```python
from build123d import *

# Parameters (mm, degrees)
SKETCH1_W           = 30
SKETCH1_H           = 150
BOSS_EXTRUDE2_DEPTH = 23
SKETCH3_W           = 28
SKETCH3_H           = 19
CUT_EXTRUDE1_DEPTH  = 193
SKETCH7_W           = 1.99467658
SKETCH7_H           = 23
BOSS_EXTRUDE4_DEPTH = 20
CUT_EXTRUDE2_DEPTH  = 20
SKETCH9_W           = 30
SKETCH9_H           = 10
BOSS_EXTRUDE5_DEPTH = 20
SKETCH11_R          = 2.5
CUT_EXTRUDE4_DEPTH  = 10
CUT_EXTRUDE5_DEPTH  = 30
FILLET1_R           = 10
SKETCH13_R          = 2.543230184
CUT_EXTRUDE6_DEPTH  = 30
FILLET2_R           = 10
FILLET3_R           = 10
FILLET4_R           = 2


with BuildPart() as part:
    # Sketch1 → Boss-Extrude2 (new body)
    with BuildSketch(Plane.XY):
        with Locations((15, 75)):
            Rectangle(SKETCH1_W, SKETCH1_H)
    extrude(amount=BOSS_EXTRUDE2_DEPTH)

    # Sketch3 → Cut-Extrude1 (cut)
    with BuildSketch(Plane(origin=(0, 150, 0), x_dir=(1, 0, 0), z_dir=(0, 1, 0))):
        with Locations((14, -11.5)):
            Rectangle(SKETCH3_W, SKETCH3_H)
    extrude(amount=-CUT_EXTRUDE1_DEPTH, mode=Mode.SUBTRACT)

    # Sketch7 → Boss-Extrude4 (add)
    with BuildSketch(Plane(origin=(0, 150, 0), x_dir=(1, 0, 0), z_dir=(0, 1, 0))):
        with Locations((29.00266171, -11.5)):
            Rectangle(SKETCH7_W, SKETCH7_H)
    extrude(amount=BOSS_EXTRUDE4_DEPTH)

    # Sketch8 → Cut-Extrude2 (cut)
    with BuildSketch(Plane(origin=(30, 0, 0), x_dir=(0, 0, -1), z_dir=(1, 0, 0))):
        with BuildLine():
            ThreePointArc((-11.5, 78), (-14.5, 75), (-11.5, 72))
            Line((-11.5, 72), (-11.5, 78))
        make_face()
        with BuildLine():
            Line((-11.5, 78), (-11.5, 72))
            ThreePointArc((-11.5, 72), (-9.378679656, 72.878679656), (-8.5, 75))
            ThreePointArc((-8.5, 75), (-9.378679656, 77.121320344), (-11.5, 78))
        make_face()
        with BuildLine():
            ThreePointArc((-13.763816566, 158.031463855), (-11.5, 157), (-9.236183434, 158.031463855))
            Line((-9.236183434, 158.031463855), (-11.5, 160))
            Line((-11.5, 160), (-13.763816566, 158.031463855))
        make_face()
        with BuildLine():
            Line((-11.5, 160), (-9.236183434, 158.031463855))
            ThreePointArc((-9.236183434, 158.031463855), (-8.690066754, 158.94915503), (-8.5, 160))
            ThreePointArc((-8.5, 160), (-8.690066754, 161.05084497), (-9.236183434, 161.968536145))
            Line((-9.236183434, 161.968536145), (-11.5, 160))
        make_face()
        with BuildLine():
            ThreePointArc((-13.763816566, 161.968536145), (-14.5, 160), (-13.763816566, 158.031463855))
            Line((-13.763816566, 158.031463855), (-11.5, 160))
            Line((-11.5, 160), (-13.763816566, 161.968536145))
        make_face()
        with BuildLine():
            Line((-11.5, 160), (-9.236183434, 161.968536145))
            ThreePointArc((-9.236183434, 161.968536145), (-11.5, 163), (-13.763816566, 161.968536145))
            Line((-13.763816566, 161.968536145), (-11.5, 160))
        make_face()
    extrude(amount=-CUT_EXTRUDE2_DEPTH, mode=Mode.SUBTRACT)

    # Sketch9 → Boss-Extrude5 (add)
    with BuildSketch(Plane.XY.offset(23)):
        with Locations((15, 75)):
            Rectangle(SKETCH9_W, SKETCH9_H)
    extrude(amount=BOSS_EXTRUDE5_DEPTH)

    # Sketch11 → Cut-Extrude4 (cut)
    with BuildSketch(Plane.XY.offset(23)):
        with Locations((7.001330855, 130)):
            Circle(SKETCH11_R)
        with Locations((7.5, 20)):
            Circle(SKETCH11_R)
    extrude(amount=-CUT_EXTRUDE4_DEPTH, mode=Mode.SUBTRACT)

    # Sketch12 → Cut-Extrude5 (cut)
    with BuildSketch(Plane.XY.offset(23)):
        Polygon((27.698367508, 150), (0, 150), (0, 140), align=None)
        Polygon((0, 0), (0, 10), (27.698367508, 0), align=None)
    extrude(amount=-CUT_EXTRUDE5_DEPTH, mode=Mode.SUBTRACT)

    # Fillet1
    fillet1_edges = [part.edges().sort_by_distance(p)[0] for p in [
        (0, 140, 1),
        (0, 10, 22),
        (0, 10, 1),
        (0, 140, 22),
    ]]
    fillet(fillet1_edges, radius=FILLET1_R)

    # Sketch13 → Cut-Extrude6 (cut)
    with BuildSketch(Plane.XY.offset(23)):
        with Locations((7.5, 20)):
            Circle(SKETCH13_R)
    extrude(amount=-CUT_EXTRUDE6_DEPTH, mode=Mode.SUBTRACT)

    # Fillet2
    fillet2_edges = [part.edges().sort_by_distance(p)[0] for p in [
        (0, 75, 43),
        (30, 75, 43),
    ]]
    fillet(fillet2_edges, radius=FILLET2_R)

    # Fillet3
    fillet3_edges = [part.edges().sort_by_distance(p)[0] for p in [
        (29.00266171, 170, 23),
        (29.00266171, 170, 0),
    ]]
    fillet(fillet3_edges, radius=FILLET3_R)

    # Fillet4
    fillet4_edges = [part.edges().sort_by_distance(p)[0] for p in [
        (30, 0, 11.5),
    ]]
    fillet(fillet4_edges, radius=FILLET4_R - 0.0001)  # a hair under: the kernel refuses the full size


solid = part.part
```
Work out the finished part from the listing and answer in its coordinate system (mm). A direction names the side the tool comes from. Coordinates: 2 decimals unless noted, no trailing zeros. Loops run counter-clockwise (first coordinate to the right, second up) from the corner with the lowest first, then second, coordinate; pieces in that order, holes last.
1) Section B-B (x = 23) is taken. Give the vertices of the cut face in (y, z).
Results:
outline: (1.7, 0) - (148.3, 0) - (148.3, 2) - (1.7, 2) - close; (1.7, 21) - (148.3, 21) - (148.3, 23) - (80, 23) - (80, 42.54) - (70, 42.54) - (70, 23) - (1.7, 23) - close
2) For faces 1 (the flat face through (14, 76, 21)), 2 (the cylindrical face through (2.85, 75.07, 39.99)), 3 (the flat face through (17.004, 3.861, 1.014)), 4 (the flat face through (15, 111, 23)), 5 (the flat face through (28.005, 158, 9)), determine the directions among +Z, -Z, +X, -X, +Y, -Y from which every point of the face is accessible in a straight line to the end or side of a thin tool.
Results:
face 1: -X, +Y, -Y
face 2: +Z, -X, +Y, -Y
face 3: +Z, -Z, -X, -Y
face 4: +Z, +X, -X, +Y
face 5: +Z, -Z, -X, +Y
3) Flat-ended cylindrical pins translate along their axes: pin 1 (16 mm diameter, centred on x = 16.5, z = 32.5, fed in from +Y); pin 2 (10 mm diameter, centred on x = 17, z = 18, fed in from +Y); pin 3 (6 mm diameter, centred on x = 17, y = 31.5, fed in from -Z); pin 4 (16 mm diameter, centred on y = 163.5, z = 11, fed in from -X). Find the tip coordinate at first contact, or state that the pin passes through.
Results:
pin 1: stops at y = 80
pin 2: stops at y = 147.58
pin 3: stops at z = 0
pin 4: stops at x = 28.01
4) Consider probe 1 along Z at (x, y) = (22.5, 130.5); probe 2 along Y at (x, z) = (7.5, 22.05); probe 3 along X at (y, z) = (130, 22.55). Determine where each line is inside the solid, lowest interval first.
Results:
probe 1: z = 0 to 2, 21 to 23
probe 2: y = 7.29 to 17.46, 22.54 to 127.55, 132.45 to 142.71
probe 3: x = 0 to 4.5, 9.5 to 30
5) Section A-A (y = 130) is taken. Give the vertices of the cut face in (x, z), plus the area to 3 significant figures.
Results:
outline: (0, 0) - (30, 0) - (30, 23) - (9.5, 23) - (9.5, 21) - (28, 21) - (28, 2) - (0, 2) - close; (0, 21) - (4.5, 21) - (4.5, 23) - (0, 23) - close
area: 148 mm2
6) For a pull along X with two mould halves and no side action, classify faces 6 (the cylindrical face through (6.68, 132.48, 22.01)), 7 (the flat face through (0, 75, 24)), 8 (the cylindrical face through (29.02, 167.15, 3.01)) as +X half, -X half, draft (parallel to the pull), parting line (faces both ways), or undercut.
Results:
face 6: undercut
face 7: -X half
face 8: draft
7) Section C-C (y = 20) is taken. Give the vertices of the cut face in (x, z).
Results:
outline: (0, 0) - (4.96, 0) - (4.96, 2) - (0, 2) - close; (0, 21) - (4.96, 21) - (4.96, 23) - (0, 23) - close; (10.04, 0) - (30, 0) - (30, 23) - (10.04, 23) - (10.04, 21) - (28, 21) - (28, 2) - (10.04, 2) - close
